Build history of the part. All positions in model axes, mm. Round coordinates to 2 decimals unless told otherwise and drop trailing zeros. Write each loop counter-clockwise with the first axis right and the second up, starting at its lowest first coordinate (ties: lowest second). Pieces come first, ordered by that corner, then holes. Notation, with made-up numbers: (56, 9.5) -> (107, 9.5) arc R19 cw to (107, 31.5) -> close; hole circle Ø4 at (-11.5, -10). An arc over 180 degrees is marked (long way). One line per question, with ' | ' between items.
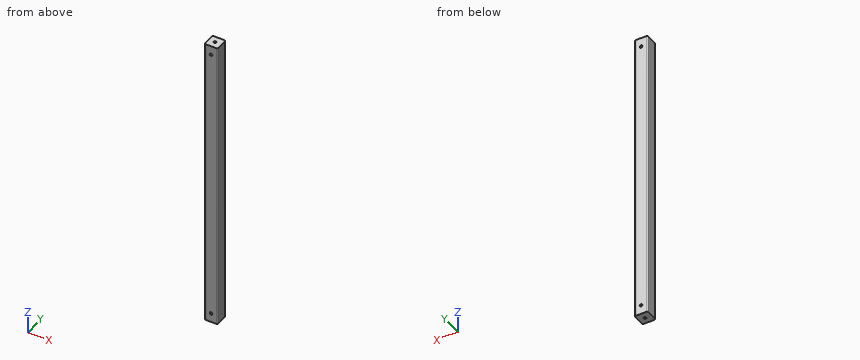
from build123d import *

# Parameters (mm, degrees)
F0_W     = 40
F0_H     = 40
F1_DEPTH = 910
F3_D     = 8
F4_R     = 4
F6_D     = 8


with BuildPart() as f1:
    # F0 (on Top) → F1 (new body)
    with BuildSketch(Plane.XY):
        Rectangle(F0_W, F0_H)
    extrude(amount=F1_DEPTH)

    # F3 (through all)
    with Locations(Plane.XY.offset(910)):
        with Locations((0, 0)):
            Hole(F3_D / 2)

    # F4
    f4_edges = [f1.edges().sort_by_distance(p)[0] for p in [
        (-20, -20, 455),
        (20, -20, 455),
        (20, 20, 455),
        (-20, 20, 455),
    ]]
    fillet(f4_edges, radius=F4_R)

    # F6 (through all)
    with Locations(Plane.XZ.offset(20)):
        with Locations((0, 27.83172), (0, 882.16828)):
            Hole(F6_D / 2)


solid = f1.part
(1) Slice it at A-A (z = 799). Write the cut outline in (x, y).
Calculated:
outline: (-20, -16) arc R4 ccw to (-16, -20) -> (16, -20) arc R4 ccw to (20, -16) -> (20, 16) arc R4 ccw to (16, 20) -> (-16, 20) arc R4 ccw to (-20, 16) -> close; hole circle Ø8 at (0, 0)
(2) Wall check: line 1 (Z direction, x = 0, y = 15); line 2 (Y direction, x = 0, z = 15); line 3 (X direction, y = -17, z = 791). Give the ranges that are in metal, low to high. Write a range as from..to.
Calculated:
line 1: 0..23.83, 31.83..878.17, 886.17..910 | line 2: -20..-4, 4..20 | line 3: -19.87..19.87
(3) Drop a flat-ended pin along its axis: pin 1 (6.5 mm diameter, centred on x = 0, y = 0, fed in from +Z). Give the stop position or say it passes through.
Calculated:
pin 1: through
